Autodesk Fusion 360 part; units mm, degrees
sketch "Sketch2" plane through (0, 0, 0) normal (1, 0, 0) x (0, 1, 0)
  line L0 (0, 0) -> (40, 0)
  line L1 (40, 0) -> (40, 30)
  line L2 (40, 30) -> (0, 30)
  line L3 (0, 30) -> (0, 0)
  line L4 (3, 3) -> (37, 3)
  line L5 (37, 3) -> (37, 27)
  line L6 (37, 27) -> (3, 27)
  line L7 (3, 27) -> (3, 3)
  line L8 (17, 3) -> (17, 18.25)
  line L9 (17, 18.25) -> (6, 18.25)
  line L10 (6, 18.25) -> (6, 15.25)
  line L11 (6, 15.25) -> (14, 15.25)
  line L12 (14, 15.25) -> (14, 3)
  line L13 (3, 14.75) -> (11, 14.75)
  line L14 (11, 14.75) -> (11, 11.75)
  line L15 (11, 11.75) -> (3, 11.75)
  line L16 (3, 11.75) -> (0, 11.75)
  line L17 (37, 11.75) -> (40, 11.75)
  line L18 (17, 12) -> (37, 13.3985)
  line L19 (17, 12.5012) -> (37, 13.8998)
  line L20 (17, 15.0012) -> (37, 17.4569)
  line L21 (17, 15.505) -> (37, 17.9607)
  line L22 (3, 3) -> (0, 3)
  line L23 (37, 3) -> (40, 3)
  dimension "d1" = -3
  dimension "d2" = 30
  dimension "d3" = 40
  dimension "d4" = 3
  dimension "d5" = 3
  dimension "d6" = 3
  dimension "d7" = 0.5
  dimension "d8" = 3
  dimension "d9" = 14
  dimension "d10" = 3
  dimension "d11" = 8.75
  dimension "d12" = 0.5
  dimension "d13" = 0.5
  dimension "d14" = 94
  dimension "d15" = 97
  dimension "d16" = 2.5
  dimension "d17" = 9
extrude "Extrude1" add sketch "Sketch2" along normal blind 18 contours L0 L1 L3 L4 L22 L23 | L1 L2 L3 L5 L6 L7 L16 L17 | L7 L13 L14 L15 | L4 L8 L9 L10 L11 L12 | L5 L8 L18 L19 | L5 L8 L20 L21
sketch "Sketch3" plane through (0, 0, 11.75) normal (0, 0, -1) x (1, 0, 0)
  line L0 (0, 0) -> (0, -11)
  line L1 (0, -11) -> (18, -11)
  line L2 (18, -11) -> (18, 0)
  line L3 (18, 0) -> (0, 0)
  line L4 (9, 0) -> (9, -6)
  line L5 (11.5, -8.5) -> (6.5, -8.5)
  line L6 (6.5, -8.5) -> (6.5, -3.5)
  line L7 (6.5, -3.5) -> (11.5, -3.5)
  line L8 (11.5, -3.5) -> (11.5, -8.5)
  line L9 (11.5, -8.5) -> (6.5, -3.5) construction
  line L10 (6.5, -8.5) -> (11.5, -3.5) construction
  point P0 (9, -6)
  dimension "d24" = 5
  dimension "d25" = 5
  dimension "d26" = 6
extrude "Extrude2" cut sketch "Sketch3" against normal blind 5 contours L5 L6 L7 L8
sketch "Sketch6" plane through (0, -1.623, 13.2184) normal (0, -0.1219, 0.9925) x (1, 0, 0)
  line L0 (0, 38.9131) -> (0, 18.7629)
  line L1 (0, 18.7629) -> (18, 18.7629)
  line L2 (18, 18.7629) -> (18, 38.9131)
  line L3 (18, 38.9131) -> (0, 38.9131)
  line L4 (0, 38.9131) -> (18, 38.9131)
  line L5 (18, 38.9131) -> (18, 18.7629)
  line L6 (18, 18.7629) -> (0, 18.7629)
  line L7 (0, 18.7629) -> (0, 38.9131)
  line L8 (1, 35.9131) -> (17, 35.9131)
  line L9 (17, 35.9131) -> (17, 21.7629)
  line L10 (17, 21.7629) -> (1, 21.7629)
  line L11 (1, 21.7629) -> (1, 35.9131)
  dimension "d34" = 1
  dimension "d35" = 1
  dimension "d36" = 3
  dimension "d37" = 3
sketch "Sketch7" plane through (0, -0.7872, 11.2574) normal (0, -0.0698, 0.9976) x (1, 0, 0)
  line L0 (0, 37.8795) -> (0, 17.8306)
  line L1 (0, 17.8306) -> (18, 17.8306)
  line L2 (18, 17.8306) -> (18, 37.8795)
  line L3 (18, 37.8795) -> (0, 37.8795)
  line L4 (0, 37.8795) -> (18, 37.8795)
  line L5 (18, 37.8795) -> (18, 17.8306)
  line L6 (18, 17.8306) -> (0, 17.8306)
  line L7 (0, 17.8306) -> (0, 37.8795)
  line L8 (1, 34.8795) -> (17, 34.8795)
  line L9 (17, 34.8795) -> (17, 20.8306)
  line L10 (17, 20.8306) -> (1, 20.8306)
  line L11 (1, 20.8306) -> (1, 34.8795)
  dimension "d38" = 1
  dimension "d39" = 1
  dimension "d40" = 3
  dimension "d41" = 3
extrude "Extrude5" cut sketch "Sketch6" against normal blind 1 contours L8 L9 L10 L11
extrude "Extrude6" cut sketch "Sketch7" against normal blind 1 contours L8 L9 L10 L11
fillet "Fillet1" radius 2.5 3 edges at (9, 0, 30) (9, 40, 30) (9, 0, 11.75)
fillet "Fillet1" radius 0.5 3 edges at (9, 3, 14.75) (9, 37, 27) (9, 3, 27)
fillet "Fillet2" radius 1 2 edges at (9, 14, 3) (9, 17, 3)
fillet "Fillet3" radius 1 2 edges at (9, 6, 18.25) (9, 17, 18.25)
sketch "Sketch4" plane through (0, 0, 3) normal (0, 0, 1) x (-1, 0, 0)
  line L0 (0, -13) -> (0, 0)
  line L1 (0, 0) -> (-18, 0)
  line L2 (-18, 0) -> (-18, -13)
  line L3 (-3.5, -10) -> (-14.5, -10)
  line L4 (-14.5, -10) -> (-14.5, 10)
  line L5 (-14.5, 10) -> (-3.5, 10)
  line L6 (-3.5, 10) -> (-3.5, -10)
  line L7 (-3.5, -10) -> (-14.5, 10) construction
  line L8 (-14.5, -10) -> (-3.5, 10) construction
  line L9 (-14.5, -10) -> (-18, -10)
  line L10 (-18, -13) -> (0, -13)
  point P0 (-9, 0)
  dimension "d27" = 11
  dimension "d28" = 20
extrude "Extrude3" cut sketch "Sketch4" against normal blind 6 contours L1 L3 L4 L6 | L1 L2 L4 L9
sketch "Sketch5" plane through (0, 0, 3) normal (0, 0, 1) x (-1, 0, 0)
  line L0 (0, -40) -> (0, -18)
  line L1 (-18, -18) -> (-18, -40)
  line L2 (-18, -40) -> (0, -40)
  line L3 (-18, -18) -> (-4, -18)
  line L4 (-4, -18) -> (-4, -40)
  line L5 (-4, -40) -> (-18, -40)
  line L6 (-18, -40) -> (-18, -18)
  line L7 (0, -18) -> (-18, -18)
  dimension "d31" = 14
extrude "Extrude4" cut sketch "Sketch5" against normal blind 5 contours L1 L2 L3 L4 L5 L6 L7
CAD build for the part. Positions are in the model's coordinates, mm. A direction names the side the tool comes from. Round coordinates to 2 decimals unless told otherwise and drop trailing zeros. Order: outer loops, then holes, each group sorted by start corner. A loop starts at its lowest first (then second) coordinate and runs counter-clockwise, first axis right, second up. Notation, with made-up numbers: (42.5, -39) - (93.5, -39) arc R21 ccw to (93.5, -10) - close; hole circle Ø7 at (-23, 69.25). An arc over 180 degrees is marked (long way). Answer as CSV lines item,"result". Start each with the question number.
1. Saw through at A-A, the plane z = 23.75. Write the cut outline in (x, y).
2. Pull direction X, two halves, no side cores. Call faces 1 (the face through (0, 15, 15)), 2 (the face through (9, 38, 11.75)), 3 (the face through (11.5, 6, 13)): +X half, -X half, draft (parallel to the pull), parting line (faces both ways), or undercut.
3. Drill centre lines: L1, parallel to Y at x = 15, z = 17; L2, parallel to Z at x = 1.5, y = 25.5; L3, parallel to Z at x = 15.5, y = 15. Where is each one in solid material? Low to high. Write a range as [from, to].
4. Tool access for faces 4 (the face through (9, 17, 16)), 5 (the face through (11, 18, 2)), 6 (the face through (9, 3.5, 13)), 7 (the face through (9.126, 17.285, 3.301)): list every direction of +Z, -Z, +X, -X, +Y, -Y with a clear straight run to the whole face (end or side of a thin tool).
5. Saw through at D-D, the plane x = 7.5. Count the separate pieces of the cut face and the enclosed holes in it, and give its area (3 significant figures).
6. Pin check, flat tips, straight feed: pin 1 (8 mm diameter, centred on x = 12, y = 29, fed in from -Z); pin 2 (1.5 mm diameter, centred on x = 12, z = 1, fed in from +Y); pin 3 (1 mm diameter, centred on x = 16, y = 13.5, fed in from -Z); pin 4 (1 mm diameter, centred on x = 10.5, z = 10, fed in from -Y). Stop position of each tip, or through.
7. Saw through at C-C, the plane y = 29.5. Write the cut outline in (x, z).
8. Saw through at B-B, the plane y = 5.5. Write the cut outline in (x, z), and give its area (4 significant figures).
Model answer:
1,outline,"(0, 0) - (18, 0) - (18, 3) - (0, 3) - close; (0, 37) - (18, 37) - (18, 40) - (0, 40) - close"
2,face 1,"-X half"
2,face 2,"draft"
2,face 3,"undercut"
3,L1,"y = [0, 3], [6, 17], [37, 40]"
3,L2,"z = [0, 3], [27, 30]"
3,L3,"z = [0, 18.25], [27, 30]"
4,face 4,"+X, -X"
4,face 5,"-Z, +X, +Y"
4,face 6,"-Z"
4,face 7,"+X, -X, +Y"
5,separate pieces,"3"
5,enclosed holes,"0"
5,area,"313 mm²"
6,pin 1,"stops at z = 27"
6,pin 2,"stops at y = 18"
6,pin 3,"stops at z = 0"
6,pin 4,"stops at y = 14"
7,outline,"(0, 0) - (4, 0) - (4, 3) - (0, 3) - close; (0, 12.87) - (1, 12.87) - (1, 13.38) - (0, 13.38) - close; (0, 16.54) - (1, 16.54) - (1, 17.04) - (0, 17.04) - close; (0, 27) - (18, 27) - (18, 30) - (0, 30) - close; (17, 12.87) - (18, 12.87) - (18, 13.38) - (17, 13.38) - close; (17, 16.54) - (18, 16.54) - (18, 17.04) - (17, 17.04) - close"
8,outline,"(0, 0) - (3.5, 0) - (3.5, 3) - (0, 3) - close; (0, 11.75) - (6.5, 11.75) - (6.5, 14.75) - (0, 14.75) - close; (0, 27) - (18, 27) - (18, 30) - (0, 30) - close; (11.5, 11.75) - (18, 11.75) - (18, 14.75) - (11.5, 14.75) - close"
8,area,"103.5 mm²"
